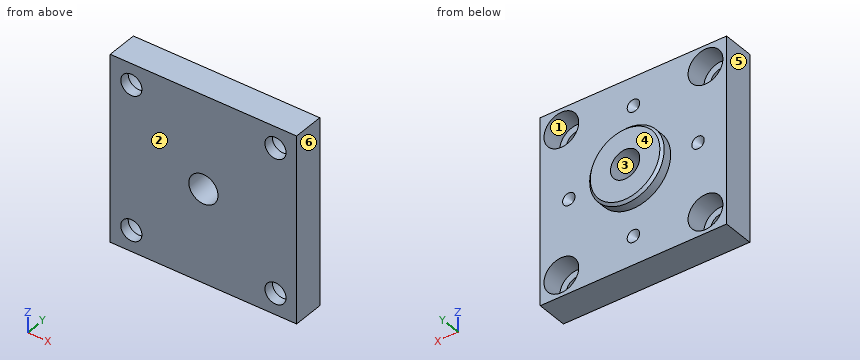
from build123d import *

# Parameters (mm, degrees)
SKETCH2_W              = 150
SKETCH2_H              = 150
BOSS_EXTRUDE1_DEPTH    = 25
SKETCH3_R              = 30
BOSS_EXTRUDE2_DEPTH    = 9
CHAMFER1_SIZE          = 2
HOLE1_D                = 17
HOLE1_CBORE_D          = 28
HOLE1_CBORE_DEPTH      = 17
M25X1_5_TAPPED_HOLE1_D = 23.5
CIRPATTERN1_COUNT      = 4


with BuildPart() as part:
    # Sketch2 → Boss-Extrude1 (new body)
    with BuildSketch(Plane(origin=(0, 0, 0), x_dir=(1, 0, 0), z_dir=(0, 1, 0))):
        Rectangle(SKETCH2_W, SKETCH2_H)
    extrude(amount=BOSS_EXTRUDE1_DEPTH)

    # Sketch3 → Boss-Extrude2 (add)
    with BuildSketch(Plane(origin=(0, 25, 0), x_dir=(1, 0, 0), z_dir=(0, 1, 0))):
        with Locations(Location((0, 0, 0), (0, 0, 270))):
            Circle(SKETCH3_R)
    extrude(amount=BOSS_EXTRUDE2_DEPTH)

    # Chamfer1
    chamfer1_edges = [part.edges().sort_by_distance(p)[0] for p in [
        (0, 34, -30),
    ]]
    chamfer(chamfer1_edges, length=CHAMFER1_SIZE)

    # Hole1 (through all)
    with Locations(Plane(origin=(0, 25, 0), x_dir=(1, 0, 0), z_dir=(0, 1, 0))):
        with Locations((-58, 58), (58, 58), (58, -58), (-58, -58)):
            CounterBoreHole(HOLE1_D / 2, HOLE1_CBORE_D / 2, HOLE1_CBORE_DEPTH)

    # Sketch13 → Cut-Revolve1 (revolve, cut)
    with BuildSketch(Plane.XY):
        Polygon((-57, 25), (-52, 20), (-52, 25), align=None)
    cut_revolve1 = revolve(axis=Axis((-52, 20, 0), (0, 1, 0)), mode=Mode.SUBTRACT)

    # M25x1.5 Tapped Hole1 (through all)
    with Locations(Plane.ZX.offset(34)):
        with Locations((0, 0)):
            Hole(M25X1_5_TAPPED_HOLE1_D / 2)

    # CirPattern1: Cut-Revolve1 ×4 about axis
    cirpattern1_axis = Axis((0, 0, 0), (0, 1, 0))
    for i in range(1, CIRPATTERN1_COUNT):
        add(cut_revolve1.rotate(cirpattern1_axis, i * 360 / CIRPATTERN1_COUNT), mode=Mode.SUBTRACT)


solid = part.part
Read the model definition and answer for the solid it produces. Units are mm, in the model's axes. Face numbers are marked on the shaded views. A direction names the side the tool comes from. Coordinates: 2 decimals unless noted, no trailing zeros. Loops run counter-clockwise (first coordinate to the right, second up) from the corner with the lowest first, then second, coordinate; pieces in that order, holes last.
Q1. The part is cut by section A-A on y = 5.5. Write down the section's boundary in (x, z).
Q2. The part is cut by section C-C on y = 27. Write down the section's boundary in (x, z), and give its area (3 significant figures).
Q3. The mould has two halves that part along X. Classify the marked faces 3, 4, 5 and 6: +X half, -X half, draft (parallel to the pull), parting line (faces both ways), or undercut.
Q4. Which of the six approach directions +Z, -Z, +X, -X, +Y, -Y give full straight-line access (tool end or side, diameter ignored) to the marked faces 1 and 2?
Q5. Each of these flat-tipped pins is pushed along its axis until it touches: pin 1 Ø22 at (x, z) = (-58, 58) entering from +Y; pin 2 Ø1.5 at (x, z) = (41, -59.5) entering from +Y; pin 3 Ø12 at (x, z) = (9.5, -33.5) entering from +Y. Where does it stop, or does it pass through?
Q6. The part is cut by section B-B on x = -61. Write down the section's boundary in (y, z).
Q7. Consider probe 1 along Z at (x, y) = (58, 2); probe 2 along X at (y, z) = (13, -58). Determine where each line is inside the solid, lowest interval first.
Results below:
1. outline: (-75, -75) - (75, -75) - (75, 75) - (-75, 75) - close; hole circle Ø17 at (-58, -58); hole circle Ø17 at (-58, 58); hole circle Ø23.5 at (0, 0); hole circle Ø17 at (58, -58); hole circle Ø17 at (58, 58)
2. outline: circle Ø60 at (0, 0); hole circle Ø23.5 at (0, 0)
2. area: 2,390 mm2
3. face 3: undercut
3. face 4: draft
3. face 5: -X half
3. face 6: +X half
4. face 1: +Y
4. face 2: +Z, -Z, +X, -X, -Y
5. pin 1: stops at y = 8
5. pin 2: stops at y = 25
5. pin 3: stops at y = 33.18
6. outline: (0, -75) - (25, -75) - (25, -71.67) - (8, -71.67) - (8, -65.95) - (0, -65.95) - close; (0, -50.05) - (8, -50.05) - (8, -44.33) - (25, -44.33) - (25, 44.33) - (8, 44.33) - (8, 50.05) - (0, 50.05) - close; (0, 65.95) - (8, 65.95) - (8, 71.67) - (25, 71.67) - (25, 75) - (0, 75) - close
7. probe 1: z = -75 to -66.5, -49.5 to 49.5, 66.5 to 75
7. probe 2: x = -75 to -72, -44 to 44, 72 to 75
